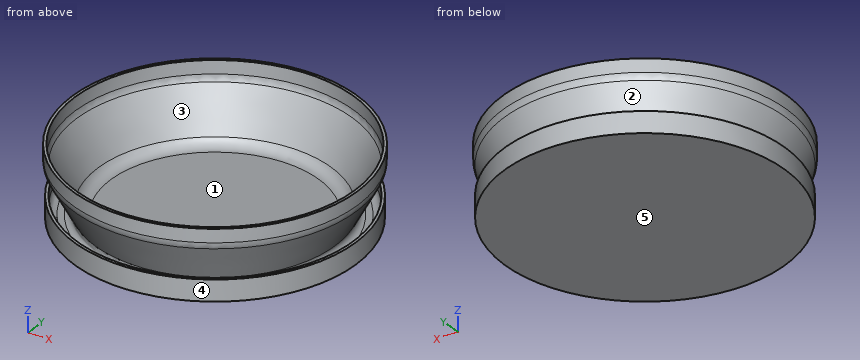
```python
from build123d import *

# Parameters (mm, degrees)
F2_R = 10


with BuildPart() as f1:
    # F0 (on Front) → F1 (revolve)
    with BuildSketch(Plane.XZ):
        with BuildLine():
            Line((0, -2), (0, 0))
            Line((0, 0), (-73.991394, 0))
            ThreePointArc((-73.991394, 0), (-79.141775, 1.428327), (-82.82087, 5.305284))
            Line((-82.82087, 5.305284), (-99.180166, 36.072645))
            Line((-99.180166, 36.072645), (-99.180166, 48))
            Line((-99.180166, 48), (-101.180166, 48))
            Line((-101.180166, 48), (-101.180166, 36))
            Line((-101.180166, 36), (-85.163954, 5.877886))
            ThreePointArc((-85.163954, 5.877886), (-85.267075, 1.939848), (-88.695744, 0))
            Line((-88.695744, 0), (-93, 0))
            ThreePointArc((-93, 0), (-96.535534, 1.464466), (-98, 5))
            Line((-98, 5), (-98, 13))
            Line((-98, 13), (-100, 13))
            Line((-100, 13), (-100, -2))
            Line((-100, -2), (0, -2))
        make_face()
    revolve(axis=Axis((0, 0, -1), (0, 0, 1)))

    # F2
    f2_edges = [f1.edges().sort_by_distance(p)[0] for p in [
        (99.180166, 0, 36.072645),
        (101.180166, 0, 36),
    ]]
    fillet(f2_edges, radius=F2_R)


solid = f1.part
```
The listing builds one solid part. Answer for the finished solid, in the listing's coordinates (mm). Face numbers are marked on the shaded views. A direction names the side the tool comes from. Round coordinates to 2 decimals unless told otherwise and drop trailing zeros. Loops run counter-clockwise (first coordinate to the right, second up) from the corner with the lowest first, then second, coordinate; pieces in that order, holes last.
Q1. Which of the six approach directions +Z, -Z, +X, -X, +Y, -Y give full straight-line access (tool end or side, diameter ignored) to the marked faces 1 and 2?
Q2. For a pull along Y with two mould halves and no side action, classify the marked faces 3, 4 and 5 as released by +Y, released by -Y, zero draft, split by the parting line, or undercut.
Q3. Given pin 1 Ø1 at (x, z) = (-13, 37) entering from -Y; pin 2 Ø3 at (x, z) = (16, 28) entering from +Y; pin 3 Ø1.5 at (x, z) = (78.5, 41) entering from -Y, each flat-ended and moving along its own axis, determine where each tip first touches the part or whether it passes through.
Q4. Find the intervals of material crossed by line 1 (Y direction, x = 33, z = 8.5); line 2 (Y direction, x = 0, z = 43.5), in increasing order.
Q5. Section A-A, the plane z = 28.5 is taken. Determine the outline of the cut face in (x, y).
Completed:
1. face 1: +Z
1. face 2: none
2. face 3: undercut
2. face 4: split by the parting line
2. face 5: zero draft
3. pin 1: stops at y = -100.32
3. pin 2: stops at y = 96.44
3. pin 3: stops at y = -64.75
4. line 1: y = -94.4 to -92.28, -80.02 to -77.81, 77.81 to 80.02, 92.28 to 94.4
4. line 2: y = -101.18 to -99.18, 99.18 to 101.18
5. outline: circle Ø194.38 at (0, 0); hole circle Ø190.31 at (0, 0)
